Design review of the part built by this model. Coordinates are the model's own, in mm. Face numbers are marked on the shaded views. A direction names the side the tool comes from. Round coordinates to 2 decimals unless told otherwise and drop trailing zeros. Order: outer loops, then holes, each group sorted by start corner. A loop starts at its lowest first (then second) coordinate and runs counter-clockwise, first axis right, second up. Notation, with made-up numbers: M -40,55.25 L -17,55.25 A18 cw -17,62.25 Z; hole C 10,-3 d5. An arc over 180 degrees is marked long. Use a Markdown table: item, result. Add a question column.
(1) Take a section at C-C (y = 25.4). Write out the cut boundary in (x, z) (1 decimal), then the cut area to 3 significant figures.
(2) For pin 1 (1.7 mm diameter, centred on y = -132.5, z = 12, fed in from +X); pin 2 (5.5 mm diameter, centred on x = 0, y = 25.4, fed in from +Z) (1 decimal); pin 3 (8.5 mm diameter, centred on x = 0, y = -63.5, fed in from +Z), all flat-tipped, find the tip position at first contact; note any pin that passes through.
(3) To check wall thickness, follow probe 1 along Y at (x, z) = (0, 12.3) (3 decimals); probe 2 along X at (y, z) = (59.5, -2.25). State the ranges of each line that lie inside material, in increasing order. Write a range as from..to.
(4) Take a section at B-B (z = -3). Write out the cut boundary in (x, y).
(5) Take a section at A-A (x = -6.5). Write out the cut boundary in (y, z).
(6) Machinability: for the marked faces 5 and 6, which of the approach directions +Z, -Z, +X, -X, +Y, -Y give a long, thin tool a straight path to every point of the face, cutting with its end or side? Answer none if there is none.
(7) The part is to be moulded in two halves that separate along X. For the marked faces 1, 2, 3 and 4, say which applies: released by +X, released by -X, zero draft, split by the parting line, or undercut.
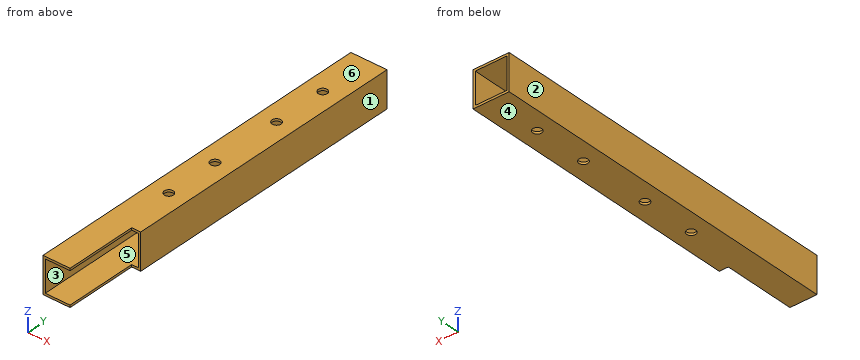
```python
from build123d import *

# Parameters (mm, degrees)
SKETCH1_W           = 25.4
SKETCH1_H           = 25.4
SKETCH1_W_2         = 22.225
SKETCH1_H_2         = 22.225
BOSS_EXTRUDE1_DEPTH = 101.6
SKETCH4_R           = 3.175
CUT_EXTRUDE3_DEPTH  = 25.4
SKETCH5_R           = 3.175
CUT_EXTRUDE4_DEPTH  = 25.4
BOSS_EXTRUDE2_DEPTH = 50.8


with BuildPart() as part:
    # Sketch1 → Boss-Extrude1 (new, symmetric)
    with BuildSketch(Plane(origin=(0, 0, 0), x_dir=(1, 0, 0), z_dir=(0, 1, 0))):
        Rectangle(SKETCH1_W, SKETCH1_H)
        Rectangle(SKETCH1_W_2, SKETCH1_H_2, mode=Mode.SUBTRACT)
    extrude(amount=BOSS_EXTRUDE1_DEPTH, both=True)

    # Sketch4 → Cut-Extrude3 (cut)
    with BuildSketch(Plane.XY.offset(12.7)):
        with Locations((0, 63.5)):
            Circle(SKETCH4_R)
        with Locations((0, -63.5)):
            Circle(SKETCH4_R)
    extrude(amount=-CUT_EXTRUDE3_DEPTH, mode=Mode.SUBTRACT)

    # Sketch5 → Cut-Extrude4 (cut)
    with BuildSketch(Plane.XY.offset(12.7)):
        with Locations((0, 25.4)):
            Circle(SKETCH5_R)
        with Locations((0, -25.4)):
            Circle(SKETCH5_R)
    extrude(amount=-CUT_EXTRUDE4_DEPTH, mode=Mode.SUBTRACT)

    # Sketch6 → Boss-Extrude2 (add)
    with BuildSketch(Plane.XZ.offset(101.6)):
        Polygon((6.35, -11.1125), (-11.1125, -11.1125), (-11.1125, 11.1125), (6.35, 11.1125), (6.35, 12.7), (-12.7, 12.7), (-12.7, -12.7), (6.35, -12.7), align=None)
    extrude(amount=BOSS_EXTRUDE2_DEPTH)


solid = part.part
```
Verdict:
| question | item | result |
|---|---|---|
| 1 | outline | M -12.7,-12.7 L -3.2,-12.7 L -3.2,-11.1 L -11.1,-11.1 L -11.1,11.1 L -3.2,11.1 L -3.2,12.7 L -12.7,12.7 Z; M 3.2,-12.7 L 12.7,-12.7 L 12.7,12.7 L 3.2,12.7 L 3.2,11.1 L 11.1,11.1 L 11.1,-11.1 L 3.2,-11.1 Z |
| 1 | area | 131 mm^2 |
| 2 | pin 1 | stops at x = 6.35 |
| 2 | pin 2 | passes through |
| 2 | pin 3 | stops at z = 12.7 |
| 3 | probe 1 | y = -152.4..-66.675, -60.325..-28.575, -22.225..22.225, 28.575..60.325, 66.675..101.6 |
| 3 | probe 2 | x = -12.7..-11.11, 11.11..12.7 |
| 4 | outline | M -12.7,-152.4 L -11.11,-152.4 L -11.11,101.6 L -12.7,101.6 Z; M 11.11,-101.6 L 12.7,-101.6 L 12.7,101.6 L 11.11,101.6 Z |
| 5 | outline | M -152.4,-12.7 L 101.6,-12.7 L 101.6,-11.11 L -152.4,-11.11 Z; M -152.4,11.11 L 101.6,11.11 L 101.6,12.7 L -152.4,12.7 Z |
| 6 | face 5 | +Y, -Y |
| 6 | face 6 | +Z, +X, -X, +Y, -Y |
| 7 | face 1 | released by +X |
| 7 | face 2 | released by -X |
| 7 | face 3 | undercut |
| 7 | face 4 | zero draft |
